The drawing under review shows one solid part. Ordinate dimensions are in mm from its lowest x, y, z. Give positions to 0.01 mm unless a question says otherwise; leave off trailing zeros. Order: outer loops, then holes, each group sorted by start corner. A loop starts at its lowest first (then second) coordinate and runs counter-clockwise, first axis right, second up. Notation, with made-up numbers: (-34.5, 43.25) - (5.5, 43.25) arc R18 ccw to (5.5, 70.25) - close; hole circle Ø11 at (-36.5, -12.5). An arc over 180 degrees is marked (long way). Use CSV: the item, a comma, the result in double quotes. Start each with the question number.
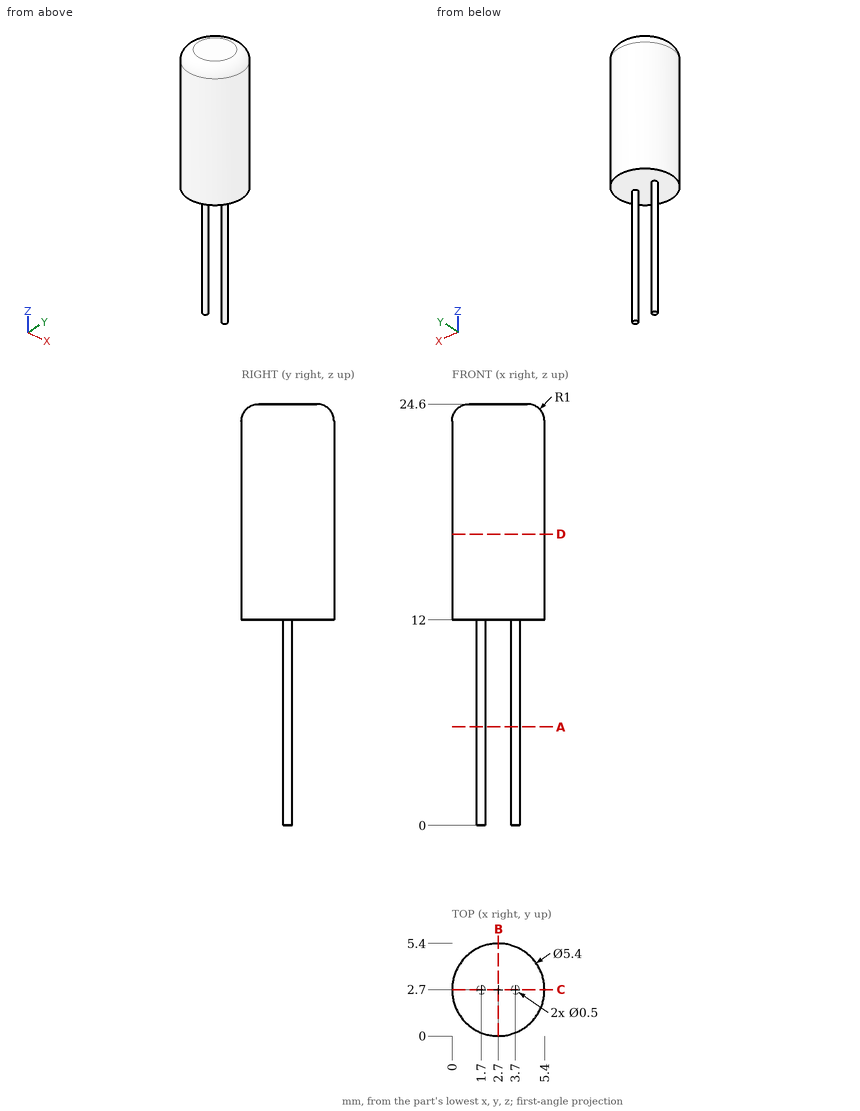
1. Consider section C-C (y = 2.7). Give the boundary of the cut face in (x, z), and give its area (3 significant figures).
2. To check wall thickness, follow L1, parallel to Z at x = 3.1, y = 4.35; L2, parallel to Z at x = 0.5, y = 1.95; L3, parallel to X at y = 3.1, z = 17. State the ranges of each line that lie inside material, in increasing order. Write a range as [from, to].
3. Consider section A-A (z = 5.75). Give the boundary of the cut face in (x, y).
4. Consider section B-B (x = 2.7). Give the boundary of the cut face in (y, z).
5. Consider section D-D (z = 17). Give the boundary of the cut face in (x, y).
6. Clearance check with flat-ended pins moving along their axes: pin 1 (2 mm diameter, centred on y = 4.5, z = 10, fed in from -X); pin 2 (2 mm diameter, centred on y = 4, z = 20.5, fed in from +X); pin 3 (1 mm diameter, centred on x = 3.5, z = 20.5, fed in from +Y). State where each tip first meets the part, or that it passes through.
Answers follow:
1,outline,"(0, 12) - (1.45, 12) - (1.45, 0) - (1.95, 0) - (1.95, 12) - (3.45, 12) - (3.45, 0) - (3.95, 0) - (3.95, 12) - (5.4, 12) - (5.4, 23.6) arc R1 ccw to (4.4, 24.6) - (1, 24.6) arc R1 ccw to (0, 23.6) - close"
1,area,"79.6 mm^2"
2,L1,"z = [12, 24.6]"
2,L2,"z = [12, 24.38]"
2,L3,"x = [0.03, 5.37]"
3,outline,"circle Ø0.5 at (1.7, 2.7); circle Ø0.5 at (3.7, 2.7)"
4,outline,"(0, 12) - (5.4, 12) - (5.4, 23.6) arc R1 ccw to (4.4, 24.6) - (1, 24.6) arc R1 ccw to (0, 23.6) - close"
5,outline,"circle Ø5.4 at (2.7, 2.7)"
6,pin 1,"passes through"
6,pin 2,"stops at x = 5.38"
6,pin 3,"stops at y = 5.38"
